Verification items for the finished model (mm, model axes). A direction names the side the tool comes from. Round coordinates to 2 decimals unless told otherwise and drop trailing zeros. Order: outer loops, then holes, each group sorted by start corner. A loop starts at its lowest first (then second) coordinate and runs counter-clockwise, first axis right, second up. Notation, with made-up numbers: (41.25, -32) -> (80.25, -32) arc R33 ccw to (80.25, 4) -> close; hole circle Ø8 at (88.25, 75.5). An arc over 180 degrees is marked (long way). Answer in a Markdown table with one row per item. Add a question column.
```python
from build123d import *

# Parameters (mm, degrees)
BOSS_EXTRUDE1_DEPTH      = 3.175
SKETCH6_R                = 5.093270322110958
BOSS_EXTRUDE2_DEPTH      = 3.175
FILLET1_R                = 0.3175
CIRPATTERN3_COUNT        = 15
FILLET1_OF_CIRPATTERN3_R = 0.3175
SKETCH7_R                = 1.27
SKETCH7_R_2              = 0.635
SKETCH7_R_3              = 0.6350000000000001
CUT_EXTRUDE1_DEPTH       = 3.175


with BuildPart() as part:
    # Sketch1 → Boss-Extrude1 (new body)
    with BuildSketch(Plane.XY):
        with BuildLine():
            Line((0.21589999999999998, 6.109270322110954), (-0.21589999999999998, 6.109270322110954))
            Line((-0.21589999999999998, 6.109270322110954), (-0.8430504444620047, 5.023013888313339))
            ThreePointArc((-0.8430504444620047, 5.023013888313339), (-0.9512218419347573, 5.003656621064491), (-1.0589504444620048, 4.981970145461529))
            ThreePointArc((-1.0589504444620048, 4.981970145461529), (-1.7e-16, 4.028486882556943), (1.0589504444620048, 4.981970145461529))
            ThreePointArc((1.0589504444620048, 4.981970145461529), (0.9512218419347568, 5.003656621064491), (0.8430504444620047, 5.023013888313339))
            Line((0.8430504444620047, 5.023013888313339), (0.21589999999999998, 6.109270322110954))
        make_face()
    boss_extrude1 = extrude(amount=BOSS_EXTRUDE1_DEPTH)

    # Sketch6 → Boss-Extrude2 (add)
    with BuildSketch(Plane.XY):
        Circle(SKETCH6_R)
    extrude(amount=BOSS_EXTRUDE2_DEPTH)

    # Fillet1
    fillet1_edges = [part.edges().sort_by_distance(p)[0] for p in [
        (-0.8430504444620048, 5.02301388831334, 1.5875),
        (-0.21589999999999998, 6.109270322110954, 1.5875),
        (0.21589999999999998, 6.109270322110954, 1.5875),
        (0.8430504444620048, 5.02301388831334, 1.5875),
    ]]
    fillet(fillet1_edges, radius=FILLET1_R)

    # CirPattern3: Boss-Extrude1 ×15 about axis
    cirpattern3_axis = Axis((0, -7e-17, 0), (0, 0, 1))
    for i in range(1, CIRPATTERN3_COUNT):
        add(boss_extrude1.rotate(cirpattern3_axis, i * 360 / CIRPATTERN3_COUNT))

    # Fillet1 of CirPattern3
    fillet1_of_cirpattern3_edges = [part.edges().sort_by_distance(p)[0] for p in [
        (-2.8132087111575306, 4.245852013620313, 1.5875),
        (-2.6820985667630595, 5.493281711035146, 1.5875),
        (-2.2876296381529846, 5.668910593515277, 1.5875),
        (-1.2728789029538499, 4.931651029068387, 1.5875),
        (-4.2969376344951105, 2.734543753417715, 1.5875),
        (-4.684537925232247, 3.92745478722371, 1.5875),
        (-4.3956073294064915, 4.248344722864849, 1.5875),
        (-3.168715924307178, 3.9875609042544276, 1.5875),
        (-5.037687004375571, 0.7504080356990912, 1.5875),
        (-5.876978118737766, 1.6825352508946705, 1.5875),
        (-5.743544580566663, 2.093201454630918, 1.5875),
        (-4.516653175467346, 2.353985273241322, 1.5875),
        (-4.907374525249817, -1.3634800486348928, 1.5875),
        (-6.053235404843441, -0.8533099156669512, 1.5875),
        (-6.098370795282413, -0.42387536124693076, 1.5875),
        (-5.083620060083269, 0.3133842031999436, 1.5875),
        (-3.928532408610401, -3.2416100457325268, 1.5875),
        (-5.182833297534428, -3.241610045732536, 1.5875),
        (-5.398733297534427, -2.8676602763784156, 1.5875),
        (-4.771582853072406, -1.7814038425808105, 1.5875),
        (-2.270411348925739, -4.559236216820256, 1.5875),
        (-3.4162722285193556, -5.069406349788216, 1.5875),
        (-3.7656057666904577, -4.815600677848326, 1.5875),
        (-3.634495622295968, -3.5681709804334942, 1.5875),
        (-0.21971554097223567, -5.088529026659036, 1.5875),
        (-1.059006655334417, -6.0206562418546286, 1.5875),
        (-1.4813707893312742, -5.930879973759519, 1.5875),
        (-1.8689710800683925, -4.737968939953519, 1.5875),
        (1.8689710800683934, -4.737968939953517, 1.5875),
        (1.4813707893312753, -5.930879973759519, 1.5875),
        (1.0590066553344182, -6.0206562418546286, 1.5875),
        (0.21971554097223658, -5.088529026659036, 1.5875),
        (3.6344956222959675, -3.5681709804334965, 1.5874999999999997),
        (3.7656057666904563, -4.815600677848327, 1.5874999999999997),
        (3.4162722285193543, -5.069406349788217, 1.5874999999999997),
        (2.270411348925738, -4.559236216820258, 1.5874999999999997),
        (4.771582853072404, -1.781403842580814, 1.5875),
        (5.398733297534425, -2.8676602763784196, 1.5875),
        (5.182833297534425, -3.24161004573254, 1.5875),
        (3.928532408610399, -3.2416100457325303, 1.5875),
        (5.083620060083269, 0.3133842031999447, 1.5875),
        (6.098370795282414, -0.42387536124692954, 1.5875),
        (6.053235404843442, -0.85330991566695, 1.5875),
        (4.907374525249819, -1.363480048634892, 1.5875),
        (4.516653175467346, 2.3539852732413205, 1.5875),
        (5.743544580566664, 2.0932014546309166, 1.5875),
        (5.8769781187377665, 1.6825352508946692, 1.5875),
        (5.037687004375571, 0.7504080356990901, 1.5875),
        (3.1687159243071803, 3.9875609042544253, 1.5875),
        (4.395607329406493, 4.2483447228648465, 1.5875),
        (4.684537925232249, 3.9274547872237076, 1.5875),
        (4.296937634495112, 2.7345437534177126, 1.5875),
        (1.2728789029538499, 4.931651029068388, 1.5875),
        (2.2876296381529846, 5.668910593515278, 1.5875),
        (2.6820985667630595, 5.493281711035147, 1.5875),
        (2.8132087111575306, 4.245852013620314, 1.5875),
    ]]
    fillet(fillet1_of_cirpattern3_edges, radius=FILLET1_OF_CIRPATTERN3_R)

    # Sketch7 → Cut-Extrude1 (cut)
    with BuildSketch(Plane.XY.offset(3.175)):
        Circle(SKETCH7_R)
        with Locations((0, 3.8099999999999996)):
            Circle(SKETCH7_R_2)
        with Locations((-3.8099999999999996, 0)):
            Circle(SKETCH7_R_3)
        with Locations(Location((3.8099999999999996, 0, 0), (0, 0, 180))):
            Circle(SKETCH7_R_3)
        with Locations(Location((-1.73e-15, -3.8099999999999996, 0), (0, 0, 180))):
            Circle(SKETCH7_R_2)
    extrude(amount=-CUT_EXTRUDE1_DEPTH, mode=Mode.SUBTRACT)


solid = part.part
```
1) Thickness scan on L1, parallel to Y at x = 0, z = 1.3 (3 decimals); L2, parallel to X at y = -1.75, z = 1.8; L3, parallel to Y at x = 4, z = 2.4. Record the ranges inside material, lowest first. Write a range as [from, to].
2) Draft check along Y on faces 4 (the face through (1.68, -5.32, 1.57)), 5 (the face through (5.079, -2.314, 1.565)), 6 (the face through (-0.17, 1.26, 1.61)), 7 (the face through (-1.3, 0.7, 0)). Enter one of: +Y half, -Y half, draft (parallel to the pull), parting line (faces both ways), or undercut.
3) Depth check by flat-ended pin: P1, Ø0.7, axis at x = 4.5, z = 2.5, coming from the -Y side; P2, Ø1, axis at x = -1, z = 0.5, coming from the +Y side. Enter the tip coordinate at first touch or a pass-through.
4) Tool access check on faces 1 (the face through (4.5, -3.242, 1.6)), 2 (the face through (3.7, -4.2, 1.6)), 3 (the face through (0.542, 5.545, 1.565)). Record the directions out of +Z, -Z, +X, -X, +Y, -Y that give a thin tool (end or side, any length) a straight path to the whole face; none if there is none.
5) Cross-section at B-B, the plane z = 2.8. Give the number of separate pieces and of enclosed holes in the cut face, and give its area (3 significant figures).
6) Cross-section at A-A, the plane y = 0. Record the boundary of the cut face in (x, z) (3 decimals).
Results below:
| question | item | result |
|---|---|---|
| 1 | L1 | [-5.093, -4.445], [-3.175, -1.27], [1.27, 3.175], [4.445, 6.109] |
| 1 | L2 | [-4.8, 4.8] |
| 1 | L3 | [-3.25, -0.61], [0.61, 4.16] |
| 2 | face 4 | -Y half |
| 2 | face 5 | undercut |
| 2 | face 6 | undercut |
| 2 | face 7 | draft |
| 3 | P1 | y = -3.24 |
| 3 | P2 | y = 5.62 |
| 4 | face 1 | +Z, -Z, +X, -Y |
| 4 | face 2 | +Z, -Z, +X |
| 4 | face 3 | +Z, -Z, +Y |
| 5 | separate pieces | 1 |
| 5 | enclosed holes | 5 |
| 5 | area | 87.4 mm² |
| 6 | outline | (-5.515, 0) -> (-4.445, 0) -> (-4.445, 3.175) -> (-5.515, 3.175) -> close; (-3.175, 0) -> (-1.27, 0) -> (-1.27, 3.175) -> (-3.175, 3.175) -> close; (1.27, 0) -> (3.175, 0) -> (3.175, 3.175) -> (1.27, 3.175) -> close; (4.445, 0) -> (5.515, 0) -> (5.515, 3.175) -> (4.445, 3.175) -> close |
